Source: CAD feature listing. Evaluate the final solid. Frame: model axes, mm. Face numbers are marked on the shaded views. A direction names the side the tool comes from. Give positions to 0.01 mm unless a question says otherwise; leave off trailing zeros. Write each loop counter-clockwise with the first axis right and the second up, starting at its lowest first coordinate (ties: lowest second). Pieces come first, ordered by that corner, then holes. Notation, with made-up numbers: (4.5, 87) -> (40.5, 87) arc R24 ccw to (40.5, 117) -> close; hole circle Ø8 at (-28, 21.5). An arc over 180 degrees is marked (long way). Write item = value, one per line.
Autodesk Fusion 360 part; units mm, degrees
sketch "Sketch1" plane through (0, 0, 0) normal (0, 1, 0) x (1, 0, 0)
  circle A0 centre (0, 0) radius 18.5
  circle A1 centre (0, 0) radius 16
  circle A2 centre (0, 0) radius 15.5 construction
  line L0 (-18.5, 0) -> (18.5, 0) construction
  circle A3 centre (15.5, 0) radius 1.5
  circle A4 centre (-15.5, 0) radius 1.5
  line L1 (9.25, -16.0215) -> (-9.25, 16.0215) construction
  line L2 (9.25, 16.0215) -> (-9.25, -16.0215) construction
  circle A5 centre (7.75, -13.4234) radius 1.5
  circle A6 centre (-7.75, -13.4234) radius 1.5
  circle A7 centre (-7.75, 13.4234) radius 1.5
  circle A8 centre (7.75, 13.4234) radius 1.5
  line L3 (-14.3875, -7) -> (14.3875, -7) construction
  circle A9 centre (0, -7) radius 3
  circle A10 centre (0, -7) radius 6
  line L4 (-1.6583, -9.5) -> (1.6583, -9.5)
  dimension "d2" = 37
  dimension "d3" = 32
  dimension "d5" = 31
  dimension "d6" = 3
  dimension "d7" = 3
  dimension "d8" = 60
  dimension "d9" = 120
  dimension "d10" = 3
  dimension "d11" = 3
  dimension "d12" = 3
  dimension "d13" = 3
  dimension "d14" = 7
  dimension "d15" = 6
  dimension "d16" = 12
  dimension "d31" = 5.5
extrude "Extrude1" add sketch "Sketch1" along normal blind 25 contours A0 | A1 A3 | A1 A3 | A1 A3 A4 A5 A6 A7 A8 | A1 A8 | A1 A8 | A1 A5 | A1 A5 | A1 A7 | A1 A7 | A1 A6 | A1 A6 | A1 A4 | A1 A4 | A9 L4 | A9 L4 | A10
extrude "Extrude2" add sketch "Sketch1" along normal blind 26 from surface at 25 contours A1 A3 | A1 A3 A4 A5 A6 A7 A8 | A1 A8 | A1 A5 | A1 A7 | A1 A6 | A1 A4 | A9 L4 | A9 L4 | A10 picked at (16.311, -0.2996) picked at (7.6973, 13.2575) picked at (8.1774, -14.1331) picked at (-8.1643, 14.1409) picked at (-7.6523, -13.282) picked at (-15.3286, 0)
extrude "Extrude3" add 1 faces at (-4.6834, 51, 2.7039) along direction (0, 1, 0) blind 15
extrude "Extrude4" add sketch "Sketch1" against normal blind 6 contours A9 L4 | A9 L4 | A10
extrude "Extrude5" add sketch "Sketch1" against normal blind 15.5 from surface at -6 contours A9 L4 | A9 L4
extrude "Extrude6" cut sketch "Sketch1" along normal blind 3.5 contours A1 A3 | A1 A3 | A1 A8 | A1 A8 | A1 A5 | A1 A5 | A1 A7 | A1 A7 | A1 A6 | A1 A6 | A1 A4 | A1 A4
extrude "Extrude7" cut sketch "Sketch1" along normal blind 12 from surface at -21.5 contours A9 L4 picked at (0.4253, -9.5717)
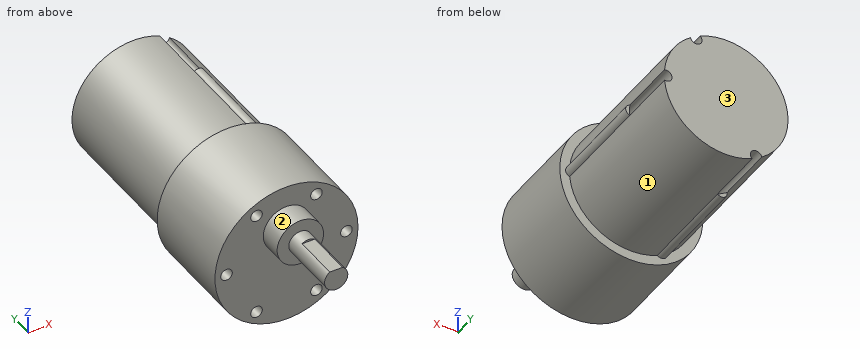
(1) Section query B-B (z = 0). Return loops of the section in (x, y), plus the area to 3 significant figures.
Values follow:
outline = (-18.5, 0) -> (-17, 0) -> (-17, 3.5) -> (-14, 3.5) -> (-14, 0) -> (14, 0) -> (14, 3.5) -> (17, 3.5) -> (17, 0) -> (18.5, 0) -> (18.5, 25) -> (17, 25) -> (17, 51) -> (16, 51) -> (16, 25) -> (14, 25) -> (14, 66) -> (-16, 66) -> (-16, 25) -> (-18.5, 25) -> close
area = 2,160 mm2
(2) Section query C-C (x = 0). Return loops of the section in (y, z).
Values follow:
outline = (-21.5, 4) -> (-6, 4) -> (-6, 1) -> (0, 1) -> (0, -18.5) -> (25, -18.5) -> (25, -16) -> (66, -16) -> (66, 16) -> (25, 16) -> (25, 18.5) -> (0, 18.5) -> (0, 13) -> (-6, 13) -> (-6, 10) -> (-9.5, 10) -> (-9.5, 9.5) -> (-21.5, 9.5) -> close
(3) First-contact query: pin 1 (3.5 mm diameter, centred on x = 8, z = 14, fed in from -Y); pin 2 (1 mm diameter, centred on y = 55.5, z = -8, fed in from -X); pin 3 (1.2 mm diameter, centred on x = 16.5, z = -0.5, fed in from +Y); pin 4 (4 mm diameter, centred on x = -7.75, z = -13.42, fed in from +Y). Flat tips, straight axial feed; report the tip coordinate or a pass-through.
Values follow:
pin_1 = 0
pin_2 = -14.13
pin_3 = 51
pin_4 = 66
(4) Access query for the marked faces 1, 2 and 3. Directions: +Z, -Z, +X, -X, +Y, -Y. A direction counts if a zero-diameter tool reaches every point of the face in a straight line with its end or side. Return the directions, or none.
Values follow:
face_1 = -Z, +Y
face_2 = -Y
face_3 = +Z, -Z, +X, -X, +Y
(5) Section query D-D (y = 55). Return loops of the section in (x, z), plus the area to 3 significant figures.
Values follow:
outline = (-9.21, -13.08) arc R1.5 cw (long way) to (-6.72, -14.52) arc R16 ccw to (15.94, -1.44) arc R1.5 cw (long way) to (15.94, 1.44) arc R16 ccw to (9.21, 13.08) arc R1.5 cw (long way) to (6.72, 14.52) arc R16 ccw to start
area = 789 mm2
(6) Material intervals for line 1 (Z direction, x = -7, y = 1); line 2 (Z direction, x = 7.75, y = 39); line 3 (Z direction, x = -7.75, y = 1.1), sorted ascending.
Values follow:
line_1 = -17.12 to -14.72, -12.12 to 12.12, 14.72 to 17.12
line_2 = -14 to 11.92, 14 to 14.92
line_3 = -16.8 to -14.92, -11.92 to 11.92, 14.92 to 16.8
